```python
from build123d import *

# Parameters (mm, degrees)
SKETCH1_W             = 203.2
SKETCH1_H             = 6.35
BOSS_EXTRUDE1_DEPTH   = 152.4
BOSS_EXTRUDE1_2_DEPTH = 152.4
SKETCH3_W             = 203.2
SKETCH3_H             = 215.9
BOSS_EXTRUDE2_DEPTH   = 0.635


with BuildPart() as part:
    # Sketch1 → Boss-Extrude1 (new body)
    with BuildSketch(Plane.XY):
        with Locations((101.6, 3.175)):
            Rectangle(SKETCH1_W, SKETCH1_H)
    extrude(amount=BOSS_EXTRUDE1_DEPTH)



with BuildPart() as body_2:
    # Sketch1 → Boss-Extrude1 2 (new body)
    with BuildSketch(Plane.XY):
        with Locations((101.6, -206.375)):
            Rectangle(SKETCH1_W, SKETCH1_H)
    extrude(amount=BOSS_EXTRUDE1_2_DEPTH)


with BuildPart() as part_1:
    add(part.part)

    add(body_2.part)  # Boss-Extrude2 merges body 2
    # Sketch3 → Boss-Extrude2 (add)
    with BuildSketch(Plane(origin=(0, 0, 0), x_dir=(-1, 0, 0), z_dir=(0, 0, -1))):
        with Locations((-101.6, -101.6)):
            Rectangle(SKETCH3_W, SKETCH3_H)
    extrude(amount=-BOSS_EXTRUDE2_DEPTH)


solid = part_1.part
```
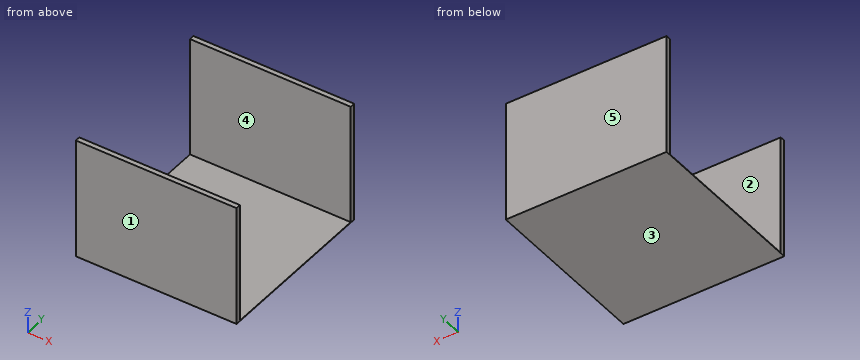
CAD build for the part. Positions are in the model's coordinates, mm. Face numbers are marked on the shaded views. A direction names the side the tool comes from. Round coordinates to 2 decimals unless told otherwise and drop trailing zeros. Order: outer loops, then holes, each group sorted by start corner. A loop starts at its lowest first (then second) coordinate and runs counter-clockwise, first axis right, second up. Notation, with made-up numbers: (-21, 6) - (-8, 6) arc R25 cw to (-8, 18) - close; hole circle Ø3 at (38.5, 44.5). An arc over 180 degrees is marked (long way). Answer in a Markdown table with one row per item. Add a question column.
(1) 3-axis set-ups, long thin cutter, end or side, ignore diameter. For the marked faces 1 and 2: which of +Z, -Z, +X, -X, +Y, -Y reach the whole face in a straight line?
(2) Mould opens along Y. For the marked faces 3, 4 and 5 say: +Y half, -Y half, draft (parallel to the pull), parting line (faces both ways), or undercut.
(3) Band-saw the part on B-B on x = 26. List the corners of the cut face in (y, z) (3 decimals).
(4) Band-saw the part on A-A on z = 61.5. List the corners of the cut face in (x, y).
(5) Band-saw the part on C-C on y = -168. List the corners of the cut face in (x, z) (3 decimals).
(6) Drop a flat-ended pin along its axis: pin 1 Ø4 at (x, y) = (134.5, -87) entering from +Z (3 decimals). Give the stop position or say it passes through.
(7) Probe L1, parallel to Y at x = 73.5, z = 52; L2, parallel to Z at x = 113, y = -184 (3 decimals). List the from-to ranges inside material, lowest first. Write a range as [from, to].
Data:
| question | item | result |
|---|---|---|
| 1 | face 1 | +Z, -Z, +X, -X, -Y |
| 1 | face 2 | +Z, +X, -X |
| 2 | face 3 | draft |
| 2 | face 4 | undercut |
| 2 | face 5 | +Y half |
| 3 | outline | (-209.55, 0) - (6.35, 0) - (6.35, 152.4) - (0, 152.4) - (0, 0.635) - (-203.2, 0.635) - (-203.2, 152.4) - (-209.55, 152.4) - close |
| 4 | outline | (0, -209.55) - (203.2, -209.55) - (203.2, -203.2) - (0, -203.2) - close; (0, 0) - (203.2, 0) - (203.2, 6.35) - (0, 6.35) - close |
| 5 | outline | (0, 0) - (203.2, 0) - (203.2, 0.635) - (0, 0.635) - close |
| 6 | pin 1 | stops at z = 0.635 |
| 7 | L1 | y = [-209.55, -203.2], [0, 6.35] |
| 7 | L2 | z = [0, 0.635] |
